Could you check a few things on this model? Use its own coordinates, in mm. A direction names the side the tool comes from. Give positions to 0.01 mm unless a question says otherwise; leave off trailing zeros. Write each loop counter-clockwise with the first axis right and the second up, starting at its lowest first coordinate (ties: lowest second). Pieces come first, ordered by that corner, then holes. Notation, with made-up numbers: M 33.25,19 L 61.25,19 A26 cw 61.25,50 Z; hole C 28,14 d11. An arc over 180 degrees is marked long. Answer as a JSON object with one key per item and string values. Group by question number.
```python
from build123d import *

# Parameters (mm, degrees)
F1_DEPTH = 25.4
F2_DEPTH = 101.6
F3_DEPTH = 838.2
F5_DEPTH = 50.8
F6_DEPTH = 76.2
F7_DEPTH = 127


with BuildPart() as f1:
    # F0 (on Top) → F1 (new body)
    with BuildSketch(Plane.XY):
        Polygon((-139.7, 12.7), (-25.4, 12.7), (-25.4, 25.4), (25.4, 25.4), (25.4, 12.7), (139.7, 12.7), (139.7, 101.6), (-139.7, 101.6), align=None)
    extrude(amount=F1_DEPTH)

    # F0 (on Top) → F2 (join)
    with BuildSketch(Plane.XY):
        Polygon((-152.4, 0), (-25.4, 0), (-25.4, 12.7), (-139.7, 12.7), (-139.7, 101.6), (-152.4, 101.6), align=None)
        Polygon((25.4, 12.7), (25.4, 0), (152.4, 0), (152.4, 101.6), (139.7, 101.6), (139.7, 12.7), align=None)
    extrude(amount=F2_DEPTH)

    # F0 (on Top) → F3 (join)
    with BuildSketch(Plane.XY):
        Polygon((-25.4, 0), (0, 0), (25.4, 0), (25.4, 12.7), (25.4, 25.4), (-25.4, 25.4), (-25.4, 12.7), align=None)
    extrude(amount=F3_DEPTH)

    # F4 (on face) → F5 (join)
    with BuildSketch(Plane(origin=(-25.4, 0, 0), x_dir=(0, -1, 0), z_dir=(-1, 0, 0))):
        with BuildLine():
            Line((-25.4, 533.4), (-25.4, 571.5))
            ThreePointArc((-25.4, 571.5), (-88.2617928475, 597.5382071525), (-114.3, 660.4))
            Line((-114.3, 660.4), (-152.4, 660.4))
            ThreePointArc((-152.4, 660.4), (-115.2025612107, 570.5974387893), (-25.4, 533.4))
        make_face()
    extrude(amount=-F5_DEPTH)



with BuildPart() as f6:
    # F4 (on face) → F6 (new body)
    with BuildSketch(Plane(origin=(-25.4, 0, 0), x_dir=(0, -1, 0), z_dir=(-1, 0, 0))):
        with BuildLine():
            ThreePointArc((0, 816.6661313275), (9.0082572424, 825.8004408344), (12.29995, 838.2))
            ThreePointArc((12.29995, 838.2), (-25.0995591656, 859.9082572424), (-25.4, 816.6661313275))
            Line((-25.4, 816.6661313275), (-25.4, 838.2))
            Line((-25.4, 838.2), (0, 838.2))
            Line((0, 838.2), (0, 816.6661313275))
        make_face()
        with BuildLine():
            Line((-25.4, 838.2), (-25.4, 816.6661313275))
            ThreePointArc((-25.4, 816.6661313275), (-12.7, 813.20005), (0, 816.6661313275))
            Line((0, 816.6661313275), (0, 838.2))
            Line((0, 838.2), (-25.4, 838.2))
        make_face()
    extrude(amount=F6_DEPTH)


with BuildPart() as f1_1:
    add(f1.part)
    # F7 (add): a face of the model
    f7_faces = [f6.part.faces().sort_by_distance(p)[0] for p in [
        (-25.4, 12.7, 838.2),
    ]]

    add(f6.part)  # F7 merges F6
    extrude(f7_faces, amount=F7_DEPTH)


solid = f1_1.part
```
1) We'd pull the mould along Z, two halves only. Please class faces 6 (the flat face through (-2, 52, 0)), 7 (the flat face through (83, 12.7, 63)), 8 (the flat face through (139.7, 58, 63)): released by +Z, released by -Z, zero draft, split by the parting line, or undercut.
2) If we section it at B-B, the plane z = 649: List the corners of the cut face in (x, y) for me.
3) For faces 1 (the flat face through (0, 133, 660.4)), 2 (the flat face through (1, 101.6, 20)), 3 (the flat face through (-82, 12.7, 63)), 4 (the flat face through (-117, 10, 101.6)), 5 (the flat face through (117, 10, 101.6)), which set-ups out of +Z, -Z, +X, -X, +Y, -Y let a thin tool reach every point of the face, with its end or its side?
4) Please list where these lines run through material, in increasing order: line 1 along X through (y, z) = (51.5, 76); line 2 along Z through (x, y) = (75.5, 87); line 3 along X through (y, z) = (93, 586.5). Write a range as from..to.
5) I'm going to push flat-ended pins straight in: pin 1 (15 mm diameter, centred on y = 7.5, z = 838.5, fed in from +X); pin 2 (3 mm diameter, centred on x = 25.5, z = 568.5, fed in from -Y); pin 3 (10 mm diameter, centred on x = -5, y = 43, fed in from +Z). Where does each tip first touch, or does it pass through?
6) If we section it at A-A, the plane x = -68.5: List the corners of the cut face in (y, z) for me.
7) If we section it at D-D, the plane z = 838.2: List the corners of the cut face in (x, y) for me.
8) If we section it at C-C, the plane x = 119.5: List the corners of the cut face in (y, z) for me.
Taken from the geometry:
{
 "1": {"face 6": "released by -Z", "face 7": "undercut", "face 8": "zero draft"},
 "2": {"outline": "M -25.4,0 L 25.4,0 L 25.4,25.4 L -25.4,25.4 Z; M -25.4,113.57 L 25.4,113.57 L 25.4,151.89 L -25.4,151.89 Z"},
 "3": {"face 1": "+Z, +X, -X, +Y", "face 2": "-Z, +X, -X, +Y", "face 3": "+Y", "face 4": "-X, +Y, -Y", "face 5": "+X, +Y, -Y"},
 "4": {"line 1": "-152.4..-139.7, 139.7..152.4", "line 2": "0..25.4", "line 3": "-25.4..25.4"},
 "5": {"pin 1": "x = 101.6", "pin 2": "y = 0", "pin 3": "z = 574.42"},
 "6": {"outline": "C 12.7,838.2 d50; M 0,0 L 101.6,0 L 101.6,25.4 L 12.7,25.4 L 12.7,101.6 L 0,101.6 Z"},
 "7": {"outline": "M -101.6,-12.3 L 101.6,-12.3 L 101.6,37.7 L -101.6,37.7 Z"},
 "8": {"outline": "M 0,0 L 101.6,0 L 101.6,25.4 L 12.7,25.4 L 12.7,101.6 L 0,101.6 Z"}
}
